Verification items for the finished model (mm, model axes). A direction names the side the tool comes from. Coordinates: 2 decimals unless noted, no trailing zeros. Write each loop counter-clockwise with the first axis right and the second up, starting at its lowest first coordinate (ties: lowest second). Pieces come first, ordered by that corner, then holes. Notation, with made-up numbers: M 31,52 L 39,52 A9 cw 39,65 Z; hole C 43,-33.5 d9. An arc over 180 degrees is marked long. One line per item, written item: value.
Autodesk Inventor part; units mm, degrees
ref_plane "YZ Plane" through (0, 0, 0) normal (1, 0, 0) x (0, 1, 0)
ref_plane "XZ Plane" through (0, 0, 0) normal (0, 1, 0) x (-1, 0, 0)
ref_plane "XY Plane" through (0, 0, 0) normal (0, 0, 1) x (1, 0, 0)
sketch "Sketch2" plane through (0, 0, 0) normal (0, 0, 1) x (1, 0, 0)
  line L0 (130.6479, 118.1756) -> (130.6479, 90.1756)
  circle A0 centre (129.6479, 104.1756) radius 14.0357
  line L1 (39.8344, 104.1756) -> (88.8344, 104.1756)
  line L2 (130.6479, 90.1756) -> (114.6267, 90.1756)
  line L3 (114.6267, 118.1756) -> (130.6479, 118.1756)
  arc A1 (143.6267, 102.9137) -> (130.6479, 118.1756) centre (129.6479, 104.1756) ccw
  arc A2 (130.6479, 90.1756) -> (143.6267, 102.9137) centre (129.6479, 104.1756) ccw
  line L4 (130.6479, 90.1756) -> (114.6267, 90.1756)
  line L5 (114.6267, 118.1756) -> (130.6479, 118.1756)
  line L6 (153.6267, 168.8936) -> (43.6267, 168.8936)
  line L7 (43.6267, 168.8936) -> (43.6267, 128.8928)
  line L8 (43.6267, 128.8928) -> (38.0267, 128.8928)
  line L9 (38.0267, 128.8928) -> (37.642, 78.8943)
  line L10 (37.642, 78.8943) -> (43.2388, 78.8943)
  line L11 (43.2388, 78.8943) -> (43.2388, 38.8936)
  line L12 (43.2388, 38.8936) -> (153.2388, 38.8936)
  line L13 (153.2388, 38.8936) -> (153.2388, 89.1756)
  line L14 (153.6267, 119.1756) -> (153.6267, 168.8936)
  line L15 (114.6267, 118.1756) -> (114.6267, 112.1756)
  line L16 (114.6267, 112.1756) -> (111.6267, 112.1756)
  line L17 (111.6267, 112.1756) -> (111.6267, 107.6756)
  line L18 (111.6267, 107.6756) -> (108.6267, 107.6756)
  line L19 (108.6267, 107.6756) -> (108.6267, 100.6756)
  line L20 (108.6267, 100.6756) -> (111.6267, 100.6756)
  line L21 (111.6267, 100.6756) -> (111.6267, 96.1756)
  line L22 (111.6267, 96.1756) -> (114.6267, 96.1756)
  line L23 (114.6267, 96.1756) -> (114.6267, 90.1756)
  line L24 (153.6267, 119.1756) -> (156.6267, 119.1756)
  line L25 (156.6267, 119.1756) -> (156.6267, 89.1756)
  line L26 (156.6267, 89.1756) -> (153.2388, 89.1756)
  circle A3 centre (129.2388, 86.6756) radius 2.15
  circle A4 centre (129.6267, 121.6756) radius 2.15
  point P0 (0, 0)
  point P1 (128.6479, 118.1756)
  point P2 (128.6479, 90.1756)
  point P3 (122.6373, 90.1756)
  point P4 (122.6373, 118.1756)
  dimension "d0" = 50
  dimension "d1" = 130
  dimension "d2" = 28.0713
  dimension "d3" = 7
  dimension "d4" = 3
  dimension "d5" = 6
  dimension "d6" = 6
  dimension "d7" = 110
  dimension "d8" = 110
  dimension "d9" = 5.6
  dimension "d10" = 3
  dimension "d11" = 32
  dimension "d13" = 10
  dimension "d14" = 30
  dimension "d15" = 3
  dimension "d18" = 28
  dimension "d28" = 4.3
  dimension "d29" = 24
  dimension "d30" = 3.5
  dimension "d31" = 4.3
  dimension "d32" = 24
  dimension "d33" = 3.5
ref_plane "Work Plane1" through (0, 0, 3) normal (0, 0, 1) x (1, 0, 0)
sketch "Sketch3" plane through (0, 0, 3) normal (0, 0, 1) x (1, 0, 0)
  circle A0 centre (56.2766, 49.819) radius 2.44
  circle A1 centre (70.2268, 49.819) radius 2.475
  circle A2 centre (83.2893, 49.819) radius 2.4
  circle A3 centre (93.7333, 49.819) radius 2.375
  circle A4 centre (104.7615, 49.819) radius 2.35
  circle A5 centre (116.1801, 49.819) radius 2.3
  circle A6 centre (127.2083, 49.819) radius 2.25
  point P0 (0, 0)
  dimension "d19" = 4.88
  dimension "d20" = 4.95
  dimension "d21" = 4.8
  dimension "d24" = 4.75
  dimension "d25" = 4.7
  dimension "d26" = 4.6
  dimension "d27" = 4.5
extrude "Extrusion3" add sketch "Sketch2" along normal blind 3
properties part number "MotorMountPlate"
Item 1: Cross-section at C-C, the plane z = 2.3. Enter the section's corners in (x, y), and give its area (3 significant figures).
The answers:
outline: M 37.64,78.89 L 43.24,78.89 L 43.24,38.89 L 153.24,38.89 L 153.24,89.18 L 156.63,89.18 L 156.63,119.18 L 153.63,119.18 L 153.63,168.89 L 43.63,168.89 L 43.63,128.89 L 38.03,128.89 Z; hole M 108.63,100.68 L 111.63,100.68 L 111.63,96.18 L 114.63,96.18 L 114.63,90.18 L 128.65,90.18 A14.04 ccw long 128.65,118.18 L 114.63,118.18 L 114.63,112.18 L 111.63,112.18 L 111.63,107.68 L 108.63,107.68 Z; hole C 129.24,86.68 d4.3; hole C 129.63,121.68 d4.3
area: 13,800 mm²
Item 2: Cross-section at B-B, the plane x = 138. Enter the section's corners in (y, z).
The answers:
outline: M 38.89,0 L 92.9,0 L 92.9,3 L 38.89,3 Z; M 115.46,0 L 168.89,0 L 168.89,3 L 115.46,3 Z
Item 3: Cross-section at D-D, the plane y = 73. Enter the section's corners in (x, z).
The answers:
outline: M 43.24,0 L 153.24,0 L 153.24,3 L 43.24,3 Z
Item 4: Cross-section at A-A, the plane y = 94.5. Enter the section's corners in (x, z).
The answers:
outline: M 37.76,0 L 114.63,0 L 114.63,3 L 37.76,3 Z; M 139.82,0 L 156.63,0 L 156.63,3 L 139.82,3 Z
Item 5: Scan lines: line 1 (X direction, y = 162, z = 2.4); line 2 (X direction, y = 45, z = 1.65); line 3 (Y direction, x = 123, z = 2.05). Record each from-to range of solid material in increasing order.
The answers:
line 1: x = 43.63 to 153.63
line 2: x = 43.24 to 153.24
line 3: y = 38.89 to 90.18, 118.18 to 168.89
Item 6: Draft check along Y on faces 1 (the face through (110, 107.676, 1)), 2 (the face through (97, 38.894, 1)), 3 (the face through (96, 105, 0)). Enter one of: released by +Y, released by -Y, zero draft, split by the parting line, or undercut.
The answers:
face 1: undercut
face 2: released by -Y
face 3: zero draft
Item 7: Access from +Z, -Z, +X, -X, +Y, -Y to the whole of each face (thin tool, end or side, straight path). Record for faces 4 (the face through (155, 89.176, 1)), 5 (the face through (41, 128.893, 1)), 6 (the face through (111.627, 98, 1)), 7 (the face through (155, 119.176, 1)).
The answers:
face 4: +Z, -Z, +X, -Y
face 5: +Z, -Z, -X, +Y
face 6: +Z, -Z
face 7: +Z, -Z, +X, +Y
Item 8: Go/stop test with flat-tipped pins: P1, Ø4, axis at x = 53, y = 99, coming from the -Z side; P2, Ø0.9, axis at x = 154.5, z = 1.5, coming from the -Y side; P3, Ø0.9, axis at y = 56.5, z = 1.5, coming from the -X side; P4, Ø1.5, axis at x = 40, z = 2, coming from the +Y side. Record where each tip stops, or that it passes through.
The answers:
P1: stops at z = 0
P2: stops at y = 89.18
P3: stops at x = 43.24
P4: stops at y = 128.89
